Could you check a few things on this drawing? It's one solid part, dimensions in mm from its lowest x, y, z. A direction names the side the tool comes from. Give positions to 0.01 mm unless a question says otherwise; leave off trailing zeros. Order: outer loops, then holes, each group sorted by start corner. A loop starts at its lowest first (then second) coordinate and runs counter-clockwise, first axis right, second up.
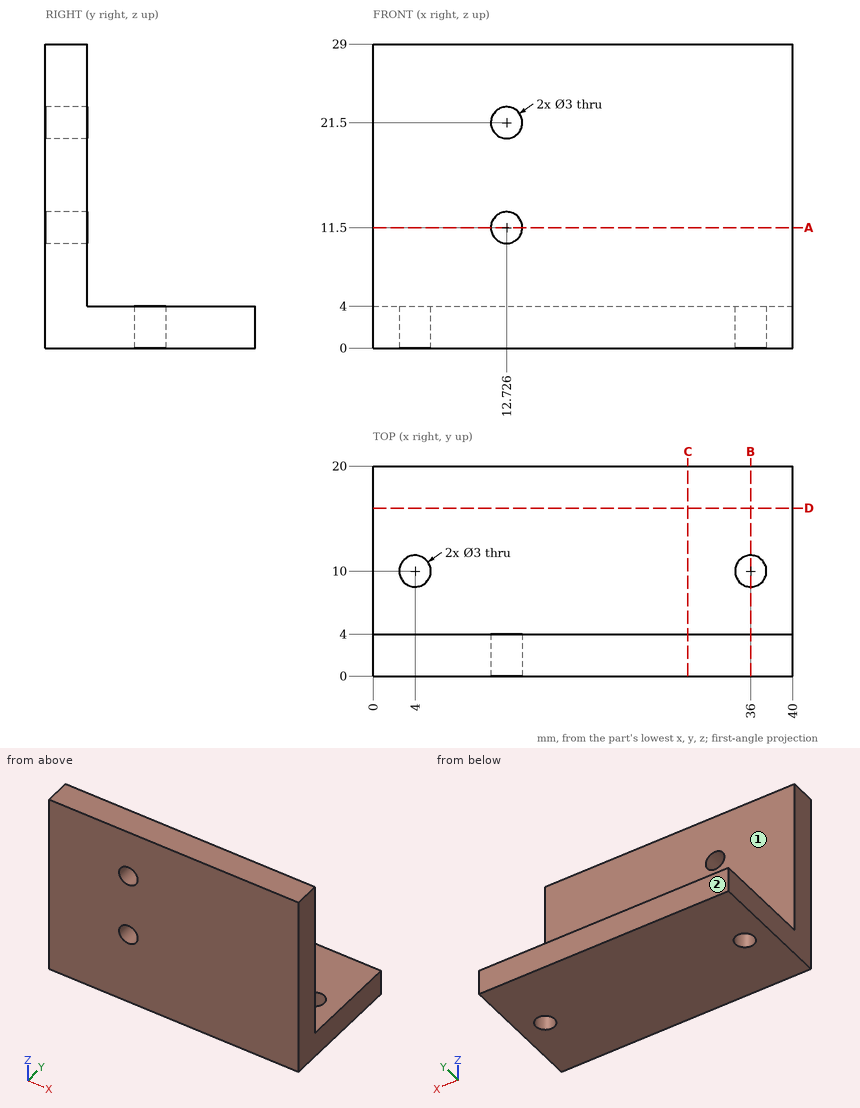
Q1. For the marked faces 1 and 2, which set-ups out of +Z, -Z, +X, -X, +Y, -Y let a thin tool reach every point of the face, with its end or its side?
Filled sheet:
face 1: +Z, +X, -X, +Y
face 2: +Z, -Z, +X, -X, +Y
Q2. I'm going to push flat-ended pins straight in: P1, Ø5, axis at x = 8.5, y = 14, coming from the +Z side; P2, Ø6, axis at x = 6, z = 12, coming from the +Y side. Where does each tip first touch, or does it pass through?
Filled sheet:
P1: stops at z = 4
P2: stops at y = 4
Q3. If we section it at C-C on x = 30: List the corners of the cut face in (y, z) for me.
Filled sheet:
outline: (0, 0) - (20, 0) - (20, 4) - (4, 4) - (4, 29) - (0, 29) - close
Q4. If we section it at D-D on y = 16: List the corners of the cut face in (x, z) for me.
Filled sheet:
outline: (0, 0) - (40, 0) - (40, 4) - (0, 4) - close
Q5. I need wall thicknesses on L1, parallel to X at y = 3.15, z = 11.5; L2, parallel to Y at x = 36, z = 2.9; L3, parallel to X at y = 9.5, z = 1.75. Which ranges of each line are inside material? Lowest first, please.
Filled sheet:
L1: x = 0 to 11.23, 14.23 to 40
L2: y = 0 to 8.5, 11.5 to 20
L3: x = 0 to 2.59, 5.41 to 34.59, 37.41 to 40
Q6. If we section it at B-B on x = 36: List the corners of the cut face in (y, z) for me, plus the area to 3 significant figures.
Filled sheet:
outline: (0, 0) - (8.5, 0) - (8.5, 4) - (4, 4) - (4, 29) - (0, 29) - close; (11.5, 0) - (20, 0) - (20, 4) - (11.5, 4) - close
area: 168 mm2
Q7. If we section it at A-A on z = 11.5: List the corners of the cut face in (x, y) for me, plus the area to 3 significant figures.
Filled sheet:
outline: (0, 0) - (11.23, 0) - (11.23, 4) - (0, 4) - close; (14.23, 0) - (40, 0) - (40, 4) - (14.23, 4) - close
area: 148 mm2
